from build123d import *

# Parameters (mm, degrees)
EXTRUDE_1_DEPTH     = 10
FILLET_1_R          = 4
EXTRUDE_2_DEPTH     = 3
SKETCH_3_R          = 1.75
CUT_EXTRUDE_1_DEPTH = 3
EXTRUDE_3_DEPTH     = 1


with BuildPart() as part:
    # Эскиз1 → Бобышка-Вытянуть1 (new body)
    with BuildSketch(Plane(origin=(0, 0, 0), x_dir=(1, 0, 0), z_dir=(0, 1, 0))):
        Polygon((-10, 0), (10, 0), (10, 20), (20, 20), (20, 18), (12, 18), (12, -2), (-12, -2), (-12, 18), (-20, 18), (-20, 20), (-10, 20), align=None)
    extrude(amount=EXTRUDE_1_DEPTH)

    # Скругление1
    fillet_1_edges = [part.edges().sort_by_distance(p)[0] for p in [
        (20, 0, -19),
        (-20, 0, -19),
        (-20, 10, -19),
        (20, 10, -19),
    ]]
    fillet(fillet_1_edges, radius=FILLET_1_R)

    # Эскиз2 → Бобышка-Вытянуть2 (add)
    with BuildSketch(Plane.XY.offset(-18)):
        with BuildLine():
            Line((-12.145, 6.703183294), (-12, 6.703183294))
            Line((-12, 6.703183294), (-12, 10))
            Line((-12, 10), (-16, 10))
            ThreePointArc((-16, 10), (-18.828427125, 8.828427125), (-20, 6))
            Line((-20, 6), (-20, 4))
            ThreePointArc((-20, 4), (-18.828427125, 1.171572875), (-16, 0))
            Line((-16, 0), (-12, 0))
            Line((-12, 0), (-12, 3.296816706))
            Line((-12, 3.296816706), (-12.145, 3.296816706))
            Line((-12.145, 3.296816706), (-15.095, 1.593633412))
            Line((-15.095, 1.593633412), (-18.045, 3.296816706))
            Line((-18.045, 3.296816706), (-18.045, 6.703183294))
            Line((-18.045, 6.703183294), (-15.095, 8.406366588))
            Line((-15.095, 8.406366588), (-12.145, 6.703183294))
        make_face()
        with BuildLine():
            Line((20, 4), (20, 6))
            ThreePointArc((20, 6), (18.828427125, 8.828427125), (16, 10))
            Line((16, 10), (12, 10))
            Line((12, 10), (12, 6.703183294))
            Line((12, 6.703183294), (12.145, 6.703183294))
            Line((12.145, 6.703183294), (15.095, 8.406366588))
            Line((15.095, 8.406366588), (18.045, 6.703183294))
            Line((18.045, 6.703183294), (18.045, 3.296816706))
            Line((18.045, 3.296816706), (15.095, 1.593633412))
            Line((15.095, 1.593633412), (12.145, 3.296816706))
            Line((12.145, 3.296816706), (12, 3.296816706))
            Line((12, 3.296816706), (12, 0))
            Line((12, 0), (16, 0))
            ThreePointArc((16, 0), (18.828427125, 1.171572875), (20, 4))
        make_face()
    extrude(amount=EXTRUDE_2_DEPTH)

    # Эскиз3 → Вырез-Вытянуть1 (cut, through all)
    with BuildSketch(Plane.XY.offset(-18)):
        with Locations((-15.095, 5)):
            Circle(SKETCH_3_R)
        with Locations((15.095, 5)):
            Circle(SKETCH_3_R)
    extrude(amount=-CUT_EXTRUDE_1_DEPTH, mode=Mode.SUBTRACT)

    # Эскиз4 → Бобышка-Вытянуть3 (add)
    with BuildSketch(Plane(origin=(0, 10, 0), x_dir=(1, 0, 0), z_dir=(0, 1, 0))):
        Polygon((-16, 15), (-12, 11), (-12, 15), align=None)
        Polygon((12, 15), (16, 15), (12, 11), align=None)
    extrude(amount=-EXTRUDE_3_DEPTH)


solid = part.part
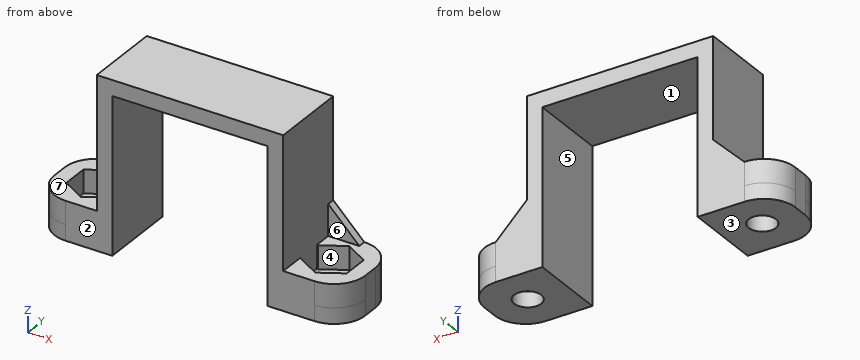
Verification items for the finished model (mm, model axes). Face numbers are marked on the shaded views. A direction names the side the tool comes from. Give positions to 0.01 mm unless a question says otherwise; leave off trailing zeros. Write each loop counter-clockwise with the first axis right and the second up, starting at its lowest first coordinate (ties: lowest second). Pieces come first, ordered by that corner, then holes.
(1) Cross-section at D-D (z = -13.5). Enter the section's corners in (x, y), plus the area to 3 significant figures.
(2) Cross-section at B-B (y = 5). Enter the section's corners in (x, z) (3 decimals), plus the area to 3 significant figures.
(3) Mould release check, pull along X, two halves, no side actions. Record for the marked faces 1 and 2: +X half, -X half, draft (parallel to the pull), parting line (faces both ways), or undercut.
(4) Cross-section at C-C (z = -18.5). Enter the section's corners in (x, y) (3 decimals), plus the area to 3 significant figures.
(5) Gauge pin test, flat ends, axial feed: pin 1 (3 mm diameter, centred on y = 5.5, z = -10, fed in from +X); pin 2 (5 mm diameter, centred on x = -5, y = 6, fed in from -Z); pin 3 (1.8 mm diameter, centred on x = -14, y = 6.5, fed in from +Z). Record the tip position at first contact, or that the pin passes through.
(6) Access from +Z, -Z, +X, -X, +Y, -Y to the whole of each face (thin tool, end or side, straight path). Record for the marked faces 3, 4, 5, 6 and 7.
(7) Material ranges on line 1 (X direction, y = 8.75, z = -5.5); line 2 (Z direction, x = -1, y = 1.75); line 3 (Z direction, x = -17, y = 6.25), recorded low to high.
(8) Cross-section at A-A (z = -5.75). Enter the section's corners in (x, y).
Worked out:
1. outline: (-14.5, 9) - (-12, 9) - (-12, 0) - (-10, 0) - (-10, 10) - (-14.5, 10) - close; (10, 0) - (12, 0) - (12, 9) - (14.5, 9) - (14.5, 10) - (10, 10) - close
1. area: 45.0 mm2
2. outline: (-20, -20) - (-16.845, -20) - (-16.845, -18) - (-18.045, -18) - (-18.045, -15) - (-20, -15) - close; (-13.345, -20) - (-10, -20) - (-10, 0) - (10, 0) - (10, -20) - (13.345, -20) - (13.345, -18) - (12, -18) - (12, 2) - (-12, 2) - (-12, -18) - (-13.345, -18) - close; (16.845, -20) - (20, -20) - (20, -15) - (18.045, -15) - (18.045, -18) - (16.845, -18) - close
2. area: 158 mm2
3. face 1: undercut
3. face 2: draft
4. outline: (-20, 4) arc R4 ccw to (-16, 0) - (-10, 0) - (-10, 10) - (-16, 10) arc R4 ccw to (-20, 6) - close; (10, 0) - (16, 0) arc R4 ccw to (20, 4) - (20, 6) arc R4 ccw to (16, 10) - (10, 10) - close; hole circle Ø3.5 at (-15.095, 5); hole circle Ø3.5 at (15.095, 5)
4. area: 167 mm2
5. pin 1: stops at x = 12
5. pin 2: stops at z = 0
5. pin 3: stops at z = -18
6. face 3: -Z, +X, -X, +Y, -Y
6. face 4: +Z
6. face 5: -Z, +Y, -Y
6. face 6: +Z, +X, -Y
6. face 7: +Z, -X, -Y
7. line 1: x = -12 to -10, 10 to 12
7. line 2: z = 0 to 2
7. line 3: z = -20 to -18
8. outline: (-12, 0) - (-10, 0) - (-10, 10) - (-12, 10) - close; (10, 0) - (12, 0) - (12, 10) - (10, 10) - close
